Can you work these out from the model? Positions are in its coordinate system, mm. A direction names the side the tool comes from. Coordinates: 2 decimals unless noted, no trailing zeros. Loops run counter-clockwise (first coordinate to the right, second up) from the corner with the lowest first, then second, coordinate; pieces in that order, holes last. Notation, with made-up numbers: (-25, 57) -> (-13, 57) arc R36 ccw to (-13, 92) -> close; hole circle Ø5 at (2.5, 51). An arc over 180 degrees is marked (long way). Put each result on its own line as item: value. Start each with the question number.
Item 1: If we section it at D-D on z = 13.5: Please give me the cut outline in (x, y), plus the area to 3 significant figures.
Item 2: If we section it at B-B on x = -49.5: Please give me the cut outline in (y, z), plus the area to 3 significant figures.
Item 3: If we section it at C-C on y = -0.95: State how many separate pieces and enclosed holes the cut face has, plus the area to 3 significant figures.
Item 4: We'd pull the mould along Z, two halves only. Please class faces 3 (the cylindrical face through (-90.882, -0.783, 9.734)), 4 (the flat face through (-49, -1.588, 12)), 5 (the cylindrical face through (-56.447, -0.195, 9.069)): pulls with the +Z half, pulls with the -Z half, needs draft (parallel to the pull), parting line crosses it, or undercut.
Item 5: If we section it at A-A on x = -13.5: Please give me the cut outline in (y, z), plus the area to 3 significant figures.
Item 6: For faces 1 (the cylindrical face through (-24.33, -0.98, 8.92)), 2 (the cylindrical face through (-50.8, -0.2, 9.58)), which set-ups out of +Z, -Z, +X, -X, +Y, -Y let a thin tool reach every point of the face, with its end or its side?
Item 7: Will these pins go through, and if not, where does the flat tip stop? P1, Ø1, axis at x = -25, z = 9.5, coming from the -Y side; P2, Ø4, axis at x = -25.5, z = 3, coming from the +Y side.
Item 8: Please list where these lines run through material, in increasing order: L1, parallel to Z at x = -20.5, y = -1.4; L2, parallel to Y at x = -53, z = 4.75; L3, parallel to Z at x = -57.5, y = -1.1. Write a range as from..to.
```python
from build123d import *

# Parameters (mm, degrees)
F1_DEPTH     = 1.5875
F2_DEPTH     = 1.18872
F0_R         = 1.5875
F3_DEPTH     = 1.5875
F0_R_2       = 1.190625
F4_DEPTH     = 0.39624
F5_DEPTH     = 1.18872
F6_T1_DEPTH  = 27.2432951274
F6_T6_DEPTH  = 16.7966475637
F6_T11_DEPTH = 16.7966475637


# Not quite as in the source:
# - a fillet or chamfer that OpenCascade refuses, or shapes differently, is made with other operations: its cross-section is extruded or revolved along the edge and cut away or added


with BuildPart() as f1:
    # F0 (on Front) → F1 (new body)
    with BuildSketch(Plane.XZ):
        with BuildLine():
            Line((-81.3593362805, 0), (-12.7, 0))
            Line((-12.7, 0), (-12.7, 1.5875))
            Line((-12.7, 1.5875), (-81.3593362805, 1.5875))
            ThreePointArc((-81.3593362805, 1.5875), (-89.2968362805, 9.525), (-81.3593362805, 17.4625))
            Line((-81.3593362805, 17.4625), (-12.7, 17.4625))
            Line((-12.7, 17.4625), (-12.7, 19.05))
            Line((-12.7, 19.05), (-81.3593362805, 19.05))
            ThreePointArc((-81.3593362805, 19.05), (-90.8843362805, 9.525), (-81.3593362805, 0))
        make_face()
    extrude(amount=F1_DEPTH)

    # F0 (on Front) → F2 (join)
    with BuildSketch(Plane.XZ):
        with BuildLine():
            Line((-81.3593362805, 1.5875), (-12.7, 1.5875))
            Line((-12.7, 1.5875), (-1.5875, 1.5875))
            Line((-1.5875, 1.5875), (-1.5875, 17.4625))
            Line((-1.5875, 17.4625), (-12.7, 17.4625))
            Line((-12.7, 17.4625), (-81.3593362805, 17.4625))
            ThreePointArc((-81.3593362805, 17.4625), (-89.2968362805, 9.525), (-81.3593362805, 1.5875))
        make_face()
        with BuildLine():
            ThreePointArc((-81.3593362805, 6.35), (-84.5343362805, 9.525), (-81.3593362805, 12.7))
            Line((-81.3593362805, 12.7), (-12.7, 12.7))
            Line((-12.7, 12.7), (-12.7, 6.35))
            Line((-12.7, 6.35), (-81.3593362805, 6.35))
        make_face(mode=Mode.SUBTRACT)
    extrude(amount=F2_DEPTH)

    # F0 (on Front) → F3 (join)
    with BuildSketch(Plane.XZ):
        with BuildLine():
            Line((-12.7, 12.7), (-81.3593362805, 12.7))
            ThreePointArc((-81.3593362805, 12.7), (-84.5343362805, 9.525), (-81.3593362805, 6.35))
            Line((-81.3593362805, 6.35), (-12.7, 6.35))
            Line((-12.7, 6.35), (-12.7, 12.7))
        make_face()
        with Locations((-81.3593362805, 9.525)):
            Circle(F0_R, mode=Mode.SUBTRACT)
        with Locations((-73.4218362805, 9.525)):
            Circle(F0_R, mode=Mode.SUBTRACT)
        with Locations((-65.4843362805, 9.525)):
            Circle(F0_R, mode=Mode.SUBTRACT)
        with Locations((-57.5468362805, 9.525)):
            Circle(F0_R, mode=Mode.SUBTRACT)
        with Locations((-49.6093362805, 9.525)):
            Circle(F0_R, mode=Mode.SUBTRACT)
        with Locations((-41.6718362805, 9.525)):
            Circle(F0_R, mode=Mode.SUBTRACT)
        with Locations((-33.7343362805, 9.525)):
            Circle(F0_R, mode=Mode.SUBTRACT)
        with Locations((-25.7968362805, 9.525)):
            Circle(F0_R, mode=Mode.SUBTRACT)
    extrude(amount=F3_DEPTH)

    # F0 (on Front) → F4 (join)
    with BuildSketch(Plane.XZ):
        with Locations((-81.3593362805, 9.525)):
            Circle(F0_R)
        with Locations((-81.3593362805, 9.525)):
            Circle(F0_R_2, mode=Mode.SUBTRACT)
        with Locations((-73.4218362805, 9.525)):
            Circle(F0_R)
        with Locations((-73.4218362805, 9.525)):
            Circle(F0_R_2, mode=Mode.SUBTRACT)
        with Locations((-65.4843362805, 9.525)):
            Circle(F0_R)
        with Locations((-65.4843362805, 9.525)):
            Circle(F0_R_2, mode=Mode.SUBTRACT)
        with Locations((-57.5468362805, 9.525)):
            Circle(F0_R)
        with Locations((-57.5468362805, 9.525)):
            Circle(F0_R_2, mode=Mode.SUBTRACT)
        with Locations((-49.6093362805, 9.525)):
            Circle(F0_R)
        with Locations((-49.6093362805, 9.525)):
            Circle(F0_R_2, mode=Mode.SUBTRACT)
        with Locations((-41.6718362805, 9.525)):
            Circle(F0_R)
        with Locations((-41.6718362805, 9.525)):
            Circle(F0_R_2, mode=Mode.SUBTRACT)
        with Locations((-33.7343362805, 9.525)):
            Circle(F0_R)
        with Locations((-33.7343362805, 9.525)):
            Circle(F0_R_2, mode=Mode.SUBTRACT)
        with Locations((-25.7968362805, 9.525)):
            Circle(F0_R)
        with Locations((-25.7968362805, 9.525)):
            Circle(F0_R_2, mode=Mode.SUBTRACT)
    extrude(amount=F4_DEPTH)

    # F0 (on Front) → F5 (join)
    with BuildSketch(Plane.XZ):
        Polygon((-12.7, 0), (0, 0), (0, 19.05), (-12.7, 19.05), (-12.7, 17.4625), (-1.5875, 17.4625), (-1.5875, 1.5875), (-12.7, 1.5875), align=None)
    extrude(amount=F5_DEPTH)

    # F6: chamfer of 1.5875 x 1.1962670545 on 3 edges, made by hand

    # F6_s2 → F6_t1 (cut)
    with BuildSketch(Plane.XY.offset(-4.0966475637)):
        Polygon((-1.5875, -1.18872), (0, 0.0075470545), (0, -1.18872), align=None)
    extrude(amount=F6_T1_DEPTH, mode=Mode.SUBTRACT)


with BuildPart() as f6_tool4:
    # F6_s5 → F6_t6 (new body)
    with BuildSketch(Plane.YZ.offset(4.0966475637)):
        Polygon((-1.18872, 17.4625), (0.0075470545, 19.05), (-1.18872, 19.05), align=None)
    extrude(amount=-F6_T6_DEPTH)

    split(bisect_by=Plane.XY.offset(17.4625), keep=Keep.TOP)


with BuildPart() as f1_1:
    add(f1.part)

    # F6_t3: cut F6_tool4
    add(f6_tool4.part, mode=Mode.SUBTRACT)


with BuildPart() as f6_tool9:
    # F6_s10 → F6_t11 (new body)
    with BuildSketch(Plane.YZ.offset(-12.7)):
        Polygon((-1.18872, 1.5875), (0.0075470545, 0), (-1.18872, 0), align=None)
    extrude(amount=F6_T11_DEPTH)

    split(bisect_by=Plane.XY.offset(1.5875), keep=Keep.BOTTOM)


with BuildPart() as f1_2:
    add(f1_1.part)

    # F6_t8: cut F6_tool9
    add(f6_tool9.part, mode=Mode.SUBTRACT)


solid = f1_2.part
```
Solutions:
1. outline: (-90.02, -1.59) -> (-88.23, -1.59) -> (-88.23, -1.19) -> (-1.59, -1.19) -> (-0.01, 0) -> (-90.02, 0) -> close
1. area: 107 mm^2
2. outline: (-1.59, 0) -> (0, 0) -> (0, 8.34) -> (-0.4, 8.34) -> (-0.4, 7.94) -> (-1.59, 7.94) -> (-1.59, 6.35) -> (-1.19, 6.35) -> (-1.19, 1.59) -> (-1.59, 1.59) -> close; (-1.59, 11.11) -> (-0.4, 11.11) -> (-0.4, 10.71) -> (0, 10.71) -> (0, 19.05) -> (-1.59, 19.05) -> (-1.59, 17.46) -> (-1.19, 17.46) -> (-1.19, 12.7) -> (-1.59, 12.7) -> close
2. area: 21.7 mm^2
3. separate pieces: 1
3. enclosed holes: 8
3. area: 1,580 mm^2
4. face 3: parting line crosses it
4. face 4: needs draft
4. face 5: undercut
5. outline: (-1.59, 0) -> (0, 0) -> (0, 19.05) -> (-1.59, 19.05) -> (-1.59, 17.46) -> (-1.19, 17.46) -> (-1.19, 12.7) -> (-1.59, 12.7) -> (-1.59, 6.35) -> (-1.19, 6.35) -> (-1.19, 1.59) -> (-1.59, 1.59) -> close
5. area: 26.4 mm^2
6. face 1: -Y
6. face 2: +Y, -Y
7. P1: y = -0.4
7. P2: y = 0
8. L1: 0..1.59, 6.35..12.7, 17.46..19.05
8. L2: -1.19..0
8. L3: 0..7.94, 11.11..19.05
